Autodesk Inventor part; units mm, degrees
ref_plane "YZ Plane" through (0, 0, 0) normal (1, 0, 0) x (0, 1, 0)
ref_plane "XZ Plane" through (0, 0, 0) normal (0, 1, 0) x (-1, 0, 0)
ref_plane "XY Plane" through (0, 0, 0) normal (0, 0, 1) x (1, 0, 0)
sketch "Sketch1" plane through (0, 0, 0) normal (0, 1, 0) x (-1, 0, 0)
  line L0 (8.2, 0) -> (19.8, 0)
  line L1 (20, -0.2) -> (20, -3.8)
  line L2 (19.8, -4) -> (10, -4)
  line L3 (10, -4) -> (10, -23.8)
  line L4 (8, -23.8) -> (8, -0.2)
  line L5 (0, 0) -> (0, -60.12)
  line L6 (9.8, -24) -> (8.2, -24)
  line L7 (20, -0.2) -> (19.8, 0)
  line L8 (20, -3.8) -> (19.8, -4)
  line L9 (8.2, 0) -> (8, -0.2)
  line L10 (8, -23.8) -> (8.2, -24)
  line L11 (9.8, -24) -> (10, -23.8)
  point P0 (8, 0)
  point P1 (20, 0)
  point P2 (20, -4)
  point P3 (10, -24)
  point P4 (8, -24)
  dimension "d0" = 40
  dimension "d1" = 4
  dimension "d2" = 20
  dimension "d6" = 10
  dimension "d7" = 2
  dimension "d8" = 20
  dimension "d9" = 16
  dimension "d10" = 0.2
  dimension "d11" = 0.2
  dimension "d12" = 0.2
  dimension "d13" = 0.2
  dimension "d14" = 0.2
  dimension "d15" = 0.2
  dimension "d16" = 0.2
  dimension "d17" = 0.2
  dimension "d18" = 0.2
  dimension "d19" = 0.2
revolve "Revolution1" add sketch "Sketch1" angle 360 about axis through (0, 0, 0) along (0, 0, -1)
sketch "Sketch2" plane through (0, 0, 0) normal (0, 0, 1) x (1, 0, 0)
  circle A0 centre (0, 0) radius 20
  point P0 (0, 16)
  dimension "d21" = 16
hole "Hole1" at (0, 16, 0) direction (0, 0, -1) diameter 3.2 end through all
pattern_circular "Circular Pattern1" count 6 over 360 about axis through (0, 0, -2) along (0, 0, -1) of "Hole1"
properties part number "TungstenFlange" material "Aluminum 6061"
Design review of the part built by this model. Coordinates are the model's own, in mm. Round coordinates to 2 decimals unless told otherwise and drop trailing zeros. Write each loop counter-clockwise with the first axis right and the second up, starting at its lowest first coordinate (ties: lowest second). Pieces come first, ordered by that corner, then holes. Notation, with made-up numbers: (5, 28.25) -> (47, 28.25) arc R30 ccw to (47, 63.25) -> close; hole circle Ø8 at (61, 82.25). An arc over 180 degrees is marked (long way). One line per item, written item: value. Start each with the question number.
Q1. Insertion check: P1, Ø4, axis at x = 5.5, z = -9, coming from the +Y side; P2, Ø4, axis at x = 13.86, y = -8, coming from the +Z side; P3, Ø4, axis at x = -13.86, y = -8, coming from the -Z side; P4, Ø13, axis at x = 0, y = 0, coming from the -Z side. Each pin has a flat end and moves straight along its axis. Give the tip position at first contact, or say it passes through.
Q2. Add section A-A (x = 0). State how many separate pieces and enclosed holes the cut face has, then the cut area to 3 significant figures.
Q3. Add section B-B (z = -20.75). Give the boundary of the cut face in (x, y), then the cut area to 3 significant figures.
Q4. The part is to be moulded in two halves that separate along X. For faces 1 (the face through (-0.07, 17.6, -2.03)), 2 (the face through (5, 9, -4)), 3 (the face through (2.17, -9.76, -14.04)), say which applies: pulls with the +X half, pulls with the -X half, needs draft (parallel to the pull), parting line crosses it, or undercut.
Q5. To check wall thickness, follow probe 1 along Y at (x, z) = (0, -13.5); probe 2 along X at (y, z) = (3, -4.25); probe 3 along Y at (x, z) = (-3, -3). State the ranges of each line that lie inside material, in increasing order.
Response:
1. P1: stops at y = 9.37
1. P2: stops at z = 0
1. P3: stops at z = -4
1. P4: passes through
2. separate pieces: 4
2. enclosed holes: 0
2. area: 150 mm^2
3. outline: circle Ø20 at (0, 0); hole circle Ø16 at (0, 0)
3. area: 113 mm^2
4. face 1: undercut
4. face 2: needs draft
4. face 3: parting line crosses it
5. probe 1: y = -10 to -8, 8 to 10
5. probe 2: x = -9.54 to -7.42, 7.42 to 9.54
5. probe 3: y = -19.77 to -7.42, 7.42 to 19.77
